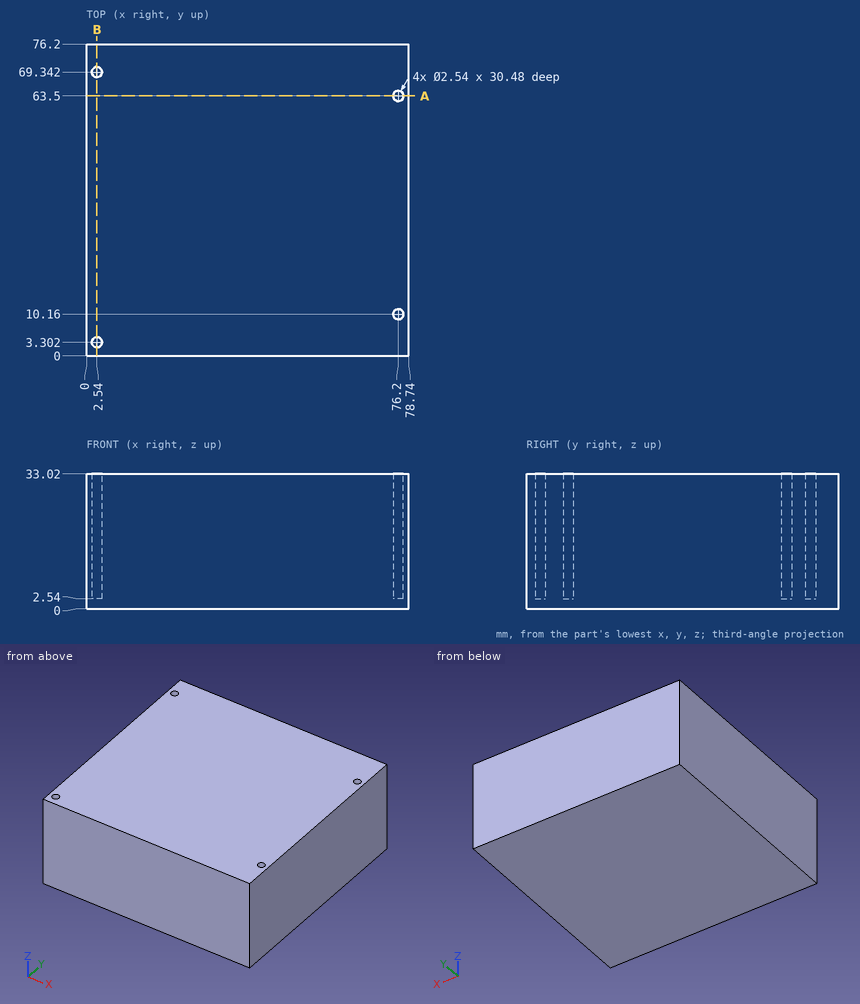
Here's the drawing with two shaded views (mm, measured from the low corner). I have some questions. Coordinates: 2 decimals unless noted, no trailing zeros. Order: outer loops, then holes, each group sorted by start corner. A loop starts at its lowest first (then second) coordinate and runs counter-clockwise, first axis right, second up. Notation, with made-up numbers: (61, -16) - (78, -16) arc R10 cw to (78, -5) - close; hole circle Ø5 at (-28, -28.75). An arc over 180 degrees is marked (long way). Answer in a Markdown table with one row per item.
1. For pin 1 (2 mm diameter, centred on x = 2.54, y = 3.302, fed in from +Z); pin 2 (3 mm diameter, centred on x = 2.5, y = 69, fed in from +Z), each with a flat end and sliding along its axis, tell me the tip position at first contact or that it passes through.
Reply:
| item | result |
|---|---|
| pin 1 | stops at z = 2.54 |
| pin 2 | stops at z = 33.02 |
2. Suppose I cut it at A-A (y = 63.5). Please give me the cut outline in (x, z), and give its area (3 significant figures).
Reply:
| item | result |
|---|---|
| outline | (0, 0) - (78.74, 0) - (78.74, 33.02) - (77.47, 33.02) - (77.47, 2.54) - (74.93, 2.54) - (74.93, 33.02) - (0, 33.02) - close |
| area | 2,520 mm^2 |
3. If I drill on line 1 along Y through (x, z) = (76, 24); line 2 along Y through (x, z) = (2, 22); line 3 along X through (y, z) = (10, 12), over which ranges is the centre line in solid material (lowest first)?
Reply:
| item | result |
|---|---|
| line 1 | y = 0 to 8.91, 11.41 to 62.25, 64.75 to 76.2 |
| line 2 | y = 0 to 2.15, 4.45 to 68.19, 70.49 to 76.2 |
| line 3 | x = 0 to 74.94, 77.46 to 78.74 |
4. Suppose I cut it at B-B (x = 2.54). Please give me the cut outline in (y, z).
Reply:
| item | result |
|---|---|
| outline | (0, 0) - (76.2, 0) - (76.2, 33.02) - (70.61, 33.02) - (70.61, 2.54) - (68.07, 2.54) - (68.07, 33.02) - (4.57, 33.02) - (4.57, 2.54) - (2.03, 2.54) - (2.03, 33.02) - (0, 33.02) - close |
